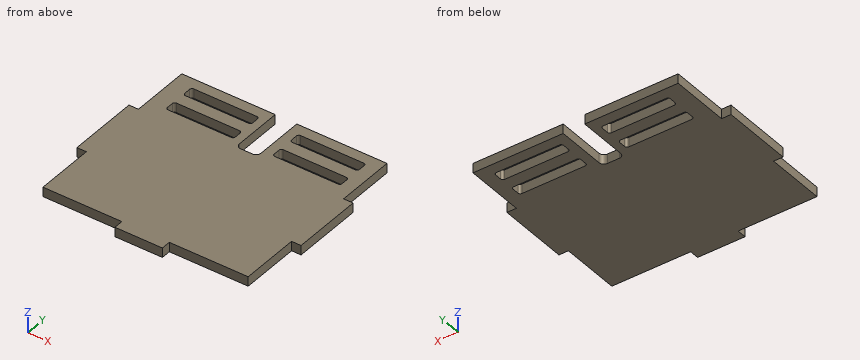
Autodesk Fusion 360 part; units mm, degrees
sketch "Sketch1" plane through (0, 0, 0) normal (0, 0, 1) x (1, 0, 0)
  line L0 (15.3385, -44.7871) -> (15.3385, -48.7871)
  line L1 (15.3385, -48.7871) -> (-4.6615, -48.7871)
  line L2 (-4.6615, -48.7871) -> (-4.6615, -44.7871)
  line L3 (-37.9015, -44.7871) -> (-4.6615, -44.7871)
  line L4 (15.3385, -44.7871) -> (48.5785, -44.7871)
  line L5 (-37.9015, -19.7871) -> (-41.9015, -19.7871)
  line L6 (-41.9015, -19.7871) -> (-41.9015, 10.2129)
  line L7 (-41.9015, 10.2129) -> (-37.9015, 10.2129)
  line L8 (-37.9015, -19.7871) -> (-37.9015, -44.7871)
  line L9 (-37.9015, 10.2129) -> (-37.9015, 35.2129)
  line L10 (48.5785, 10.2129) -> (52.5785, 10.2129)
  line L11 (52.5785, 10.2129) -> (52.5785, -19.7871)
  line L12 (52.5785, -19.7871) -> (48.5785, -19.7871)
  line L13 (48.5785, -19.7871) -> (48.5785, -21.9637)
  line L14 (48.5785, -21.9637) -> (48.5785, -44.7871)
  line L15 (48.5785, 10.2129) -> (48.5785, 13.5404)
  line L16 (48.5785, 13.5404) -> (48.5785, 35.2129)
  line L17 (-29.5277, 30.6619) -> (-2.944, 30.6619)
  line L18 (-1.944, 29.6619) -> (-1.944, 26.8722)
  line L19 (-2.944, 25.8722) -> (-29.5277, 25.8722)
  line L20 (-30.5277, 26.8722) -> (-30.5277, 29.6619)
  arc A0 (-30.5277, 26.8722) -> (-29.5277, 25.8722) centre (-29.5277, 26.8722) ccw
  arc A1 (-29.5277, 30.6619) -> (-30.5277, 29.6619) centre (-29.5277, 29.6619) ccw
  arc A2 (-1.944, 29.6619) -> (-2.944, 30.6619) centre (-2.944, 29.6619) ccw
  arc A3 (-2.944, 25.8722) -> (-1.944, 26.8722) centre (-2.944, 26.8722) ccw
  line L21 (-30.5277, 16.8722) -> (-30.5277, 19.6619)
  line L22 (-29.5277, 20.6619) -> (-2.944, 20.6619)
  arc A4 (-1.944, 19.6619) -> (-2.944, 20.6619) centre (-2.944, 19.6619) ccw
  line L23 (-1.944, 19.6619) -> (-1.944, 16.8722)
  arc A5 (-29.5277, 20.6619) -> (-30.5277, 19.6619) centre (-29.5277, 19.6619) ccw
  arc A6 (-2.944, 15.8722) -> (-1.944, 16.8722) centre (-2.944, 16.8722) ccw
  arc A7 (-30.5277, 16.8722) -> (-29.5277, 15.8722) centre (-29.5277, 16.8722) ccw
  line L24 (-2.944, 15.8722) -> (-29.5277, 15.8722)
  arc A8 (42.056, 25.8722) -> (43.056, 26.8722) centre (42.056, 26.8722) ccw
  line L25 (42.056, 25.8722) -> (15.4723, 25.8722)
  line L26 (14.4723, 26.8722) -> (14.4723, 29.6619)
  arc A9 (14.4723, 16.8722) -> (15.4723, 15.8722) centre (15.4723, 16.8722) ccw
  arc A10 (15.4723, 20.6619) -> (14.4723, 19.6619) centre (15.4723, 19.6619) ccw
  arc A11 (42.056, 15.8722) -> (43.056, 16.8722) centre (42.056, 16.8722) ccw
  arc A12 (43.056, 19.6619) -> (42.056, 20.6619) centre (42.056, 19.6619) ccw
  arc A13 (15.4723, 30.6619) -> (14.4723, 29.6619) centre (15.4723, 29.6619) ccw
  line L27 (42.056, 15.8722) -> (15.4723, 15.8722)
  line L28 (43.056, 29.6619) -> (43.056, 26.8722)
  arc A14 (14.4723, 26.8722) -> (15.4723, 25.8722) centre (15.4723, 26.8722) ccw
  line L29 (43.056, 19.6619) -> (43.056, 16.8722)
  line L30 (15.4723, 30.6619) -> (42.056, 30.6619)
  line L31 (14.4723, 16.8722) -> (14.4723, 19.6619)
  line L32 (15.4723, 20.6619) -> (42.056, 20.6619)
  arc A15 (43.056, 29.6619) -> (42.056, 30.6619) centre (42.056, 29.6619) ccw
  line L33 (10.5491, 35.2129) -> (10.5491, 14.5299)
  line L34 (8.5491, 12.5299) -> (3.4812, 12.5299)
  line L35 (1.4812, 14.5299) -> (1.4812, 35.2129)
  arc A16 (1.4812, 14.5299) -> (3.4812, 12.5299) centre (3.4812, 14.5299) ccw
  arc A17 (8.5491, 12.5299) -> (10.5491, 14.5299) centre (8.5491, 14.5299) ccw
  line L36 (10.5491, 35.2129) -> (48.5785, 35.2129)
  line L37 (1.4812, 35.2129) -> (-37.9015, 35.2129)
extrude "Extrude1" add sketch "Sketch1" along normal blind 4
Read the model definition and answer for the solid it produces. Units are mm, in the model's axes. Coordinates: 2 decimals unless noted, no trailing zeros. Loops run counter-clockwise (first coordinate to the right, second up) from the corner with the lowest first, then second, coordinate; pieces in that order, holes last.
Q1. Each of these flat-tipped pins is pushed along its axis until it touches: pin 1 Ø2 at (x, z) = (-28, 2.5) entering from -Y; pin 2 Ø1.4 at (y, z) = (17.5, 2) entering from +X; pin 3 Ø0.8 at (y, z) = (28.5, 2.5) entering from -X. Where does it stop, or does it pass through?
Q2. The part is cut by section C-C on z = 3.3. Give the number of separate pieces and of enclosed holes in the cut face, and give its area (3 significant figures).
Q3. Consider probe 1 along Y at (x, z) = (-16, 0.45); probe 2 along Y at (x, z) = (-3, 1.7); probe 3 along X at (y, z) = (32.5, 2.85). Determine where each line is inside the solid, lowest interval first.
Q4. The part is cut by section B-B on y = -39.5. Write down the section's boundary in (x, z), and give its area (3 significant figures).
Q5. The part is cut by section A-A on x = -24. Write down the section's boundary in (y, z).
Results below:
1. pin 1: stops at y = -44.79
1. pin 2: stops at x = 48.58
1. pin 3: stops at x = -37.9
2. separate pieces: 1
2. enclosed holes: 4
2. area: 6,490 mm2
3. probe 1: y = -44.79 to 15.87, 20.66 to 25.87, 30.66 to 35.21
3. probe 2: y = -48.79 to 15.87, 20.66 to 25.87, 30.66 to 35.21
3. probe 3: x = -37.9 to 1.48, 10.55 to 48.58
4. outline: (-37.9, 0) - (48.58, 0) - (48.58, 4) - (-37.9, 4) - close
4. area: 346 mm2
5. outline: (-44.79, 0) - (15.87, 0) - (15.87, 4) - (-44.79, 4) - close; (20.66, 0) - (25.87, 0) - (25.87, 4) - (20.66, 4) - close; (30.66, 0) - (35.21, 0) - (35.21, 4) - (30.66, 4) - close
